Design review of the part built by this model. Coordinates are the model's own, in mm. Face numbers are marked on the shaded views. Coordinates: 2 decimals unless noted, no trailing zeros. Loops run counter-clockwise (first coordinate to the right, second up) from the corner with the lowest first, then second, coordinate; pieces in that order, holes last. Notation, with made-up numbers: (-20, 73.5) -> (13, 73.5) arc R24 cw to (13, 93.5) -> close; hole circle Ø1 at (-16.5, 68). An arc over 180 degrees is marked (long way). Answer in a Markdown table with one row per item.
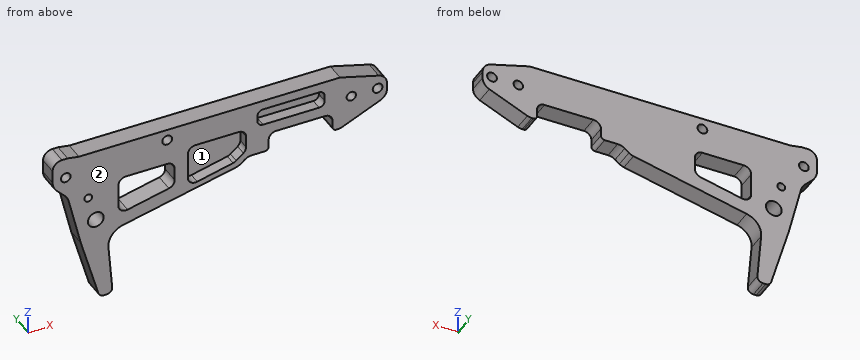
```python
from build123d import *

# Parameters (mm, degrees)
SKETCH1_R           = 2.6
SKETCH1_R_2         = 2.1
SKETCH1_R_3         = 4.2
SKETCH1_R_4         = 2.5
BOSS_EXTRUDE1_DEPTH = 10
FILLET2_R           = 6
FILLET3_R           = 3
CUT_EXTRUDE1_DEPTH  = 11
SKETCH7_R           = 2.6
CUT_EXTRUDE4_DEPTH  = 11
FILLET8_R           = 5
FILLET9_R           = 4
SKETCH10_W          = 34
SKETCH10_H          = 10
CUT_EXTRUDE6_DEPTH  = 11
FILLET10_R          = 4
CUT_EXTRUDE7_DEPTH  = 6
FILLET14_R          = 6
FILLET15_R          = 2
FILLET16_R          = 10
FILLET17_R          = 8
FILLET18_R          = 4
SKETCH13_W          = 35.854861743
SKETCH13_H          = 9
CUT_EXTRUDE8_DEPTH  = 6
FILLET19_R          = 3


with BuildPart() as part:
    # Sketch1 → Boss-Extrude1 (new body)
    with BuildSketch(Plane(origin=(0, 0, 0), x_dir=(1, 0, 0), z_dir=(0, 1, 0))):
        Polygon((164, 19), (139, 30), (90, 30), (85, 34), (15, 50), (18, 86), (11, 86), (1, 51), (-6, 22), (-14, 14), (-14, 2), (-14, -1), (-6, -1), (0, 0), (139, 0), (164, 7), align=None)
        with Locations((-7, 10)):
            Circle(SKETCH1_R, mode=Mode.SUBTRACT)
        with Locations((159, 13)):
            Circle(SKETCH1_R, mode=Mode.SUBTRACT)
        with Locations((5, 26)):
            Circle(SKETCH1_R_2, mode=Mode.SUBTRACT)
        with Locations((9, 40)):
            Circle(SKETCH1_R_3, mode=Mode.SUBTRACT)
        with Locations((145, 13)):
            Circle(SKETCH1_R_4, mode=Mode.SUBTRACT)
    extrude(amount=BOSS_EXTRUDE1_DEPTH)

    # Fillet2
    fillet2_edges = [part.edges().sort_by_distance(p)[0] for p in [
        (139, 5, -30),
        (164, 5, -19),
        (164, 5, -7),
    ]]
    fillet(fillet2_edges, radius=FILLET2_R)

    # Fillet3
    fillet3_edges = [part.edges().sort_by_distance(p)[0] for p in [
        (11, 5, -86),
        (18, 5, -86),
    ]]
    fillet(fillet3_edges, radius=FILLET3_R)

    # Sketch4 → Cut-Extrude1 (cut, through all)
    with BuildSketch(Plane(origin=(0, 10, 0), x_dir=(1, 0, 0), z_dir=(0, 1, 0))):
        Polygon((21, 41), (21, 20), (51, 20), (51, 34), align=None)
    extrude(amount=-CUT_EXTRUDE1_DEPTH, mode=Mode.SUBTRACT)

    # Sketch7 → Cut-Extrude4 (cut, through all)
    with BuildSketch(Plane(origin=(0, 10, 0), x_dir=(1, 0, 0), z_dir=(0, 1, 0))):
        with Locations((47, 6)):
            Circle(SKETCH7_R)
    extrude(amount=-CUT_EXTRUDE4_DEPTH, mode=Mode.SUBTRACT)

    # Fillet8
    fillet8_edges = [part.edges().sort_by_distance(p)[0] for p in [
        (-14, 5, 1),
    ]]
    fillet(fillet8_edges, radius=FILLET8_R)

    # Fillet9
    fillet9_edges = [part.edges().sort_by_distance(p)[0] for p in [
        (21, 5, -41),
        (51, 5, -34),
        (51, 5, -20),
        (21, 5, -20),
    ]]
    fillet(fillet9_edges, radius=FILLET9_R)

    # Sketch10 → Cut-Extrude6 (cut, through all)
    with BuildSketch(Plane(origin=(0, 10, 0), x_dir=(1, 0, 0), z_dir=(0, 1, 0))):
        with Locations((118, 25)):
            Rectangle(SKETCH10_W, SKETCH10_H)
    extrude(amount=-CUT_EXTRUDE6_DEPTH, mode=Mode.SUBTRACT)

    # Fillet10
    fillet10_edges = [part.edges().sort_by_distance(p)[0] for p in [
        (135, 5, -20),
        (101, 5, -20),
    ]]
    fillet(fillet10_edges, radius=FILLET10_R)

    # Sketch12 → Cut-Extrude7 (cut)
    with BuildSketch(Plane(origin=(0, 0, 0), x_dir=(1, 0, 0), z_dir=(0, 1, 0))):
        Polygon((58, 37), (83, 31.034746853), (89, 26.034746853), (89, 14), (58, 14), align=None)
    extrude(amount=CUT_EXTRUDE7_DEPTH, mode=Mode.SUBTRACT)

    # Fillet14
    fillet14_edges = [part.edges().sort_by_distance(p)[0] for p in [
        (85, 5, -34),
        (90, 5, -30),
    ]]
    fillet(fillet14_edges, radius=FILLET14_R)

    # Fillet15
    fillet15_edges = [part.edges().sort_by_distance(p)[0] for p in [
        (101, 5, -30),
        (135, 5, -30),
    ]]
    fillet(fillet15_edges, radius=FILLET15_R)

    # Fillet16
    fillet16_edges = [part.edges().sort_by_distance(p)[0] for p in [
        (15, 5, -50),
    ]]
    fillet(fillet16_edges, radius=FILLET16_R)

    # Fillet17
    fillet17_edges = [part.edges().sort_by_distance(p)[0] for p in [
        (-14, 5, -14),
        (-6, 5, -22),
    ]]
    fillet(fillet17_edges, radius=FILLET17_R)

    # Fillet18
    fillet18_edges = [part.edges().sort_by_distance(p)[0] for p in [
        (58, 3, -37),
        (58, 3, -14),
        (89, 3, -14),
        (89, 3, -26.034746853),
        (83, 3, -31.034746853),
    ]]
    fillet(fillet18_edges, radius=FILLET18_R)

    # Sketch13 → Cut-Extrude8 (cut)
    with BuildSketch(Plane.XZ):
        with Locations((112.927430872, -9.5)):
            Rectangle(SKETCH13_W, SKETCH13_H)
    extrude(amount=-CUT_EXTRUDE8_DEPTH, mode=Mode.SUBTRACT)

    # Fillet19
    fillet19_edges = [part.edges().sort_by_distance(p)[0] for p in [
        (130.854861743, 3, -5),
        (130.854861743, 3, -14),
        (95, 3, -14),
        (95, 3, -5),
    ]]
    fillet(fillet19_edges, radius=FILLET19_R)


solid = part.part
```
(1) To check wall thickness, follow probe 1 along X at (y, z) = (5.25, -26); probe 2 along X at (y, z) = (2.25, -13); probe 3 along X at (y, z) = (4.5, -10). State the ranges of each line that lie inside material, in increasing order.
Evaluation:
| item | result |
|---|---|
| probe 1 | x = -5.03 to 2.9, 7.1 to 21, 51 to 58, 88.55 to 101, 135 to 148.09 |
| probe 2 | x = -13.66 to 95.76, 130.09 to 142.5, 147.5 to 156.4, 161.6 to 164 |
| probe 3 | x = -14 to -9.6, -4.4 to 95, 130.85 to 163.8 |
(2) Take a section at A-A on y = 2.5. Count the separate pieces of the cut face and the enclosed holes in it, and give its area (3 significant figures).
Evaluation:
| item | result |
|---|---|
| separate pieces | 1 |
| enclosed holes | 9 |
| area | 4,700 mm² |
(3) For pin 1 (3 mm diameter, centred on y = 3, z = -20, fed in from -X); pin 2 (5 mm diameter, centred on x = 107, y = 4, fed in from -Z); pin 3 (1 mm diameter, centred on y = 9, z = -51.5, fed in from +X); pin 4 (7 mm diameter, centred on x = 159, z = -13, fed in from -Y), all flat-tipped, find the tip position at first contact; note any pin that passes through.
Evaluation:
| item | result |
|---|---|
| pin 1 | stops at x = -9.5 |
| pin 2 | stops at z = -20.03 |
| pin 3 | stops at x = 18.37 |
| pin 4 | stops at y = 0 |
(4) Take a section at C-C on z = -68.5. Give the boundary of the cut face in (x, y).
Evaluation:
| item | result |
|---|---|
| outline | (6, 0) -> (16.54, 0) -> (16.54, 10) -> (6, 10) -> close |
(5) Draft analysis for pull direction X (two halves, no side actions). For the marked faces 1 and 2, state which applies: pulls with the +X half, pulls with the -X half, needs draft (parallel to the pull), parting line crosses it, or undercut.
Evaluation:
| item | result |
|---|---|
| face 1 | undercut |
| face 2 | needs draft |
(6) Take a section at B-B on x = 108. Give the boundary of the cut face in (y, z), and give its area (3 significant figures).
Evaluation:
| item | result |
|---|---|
| outline | (0, -20) -> (10, -20) -> (10, 0) -> (0, 0) -> (0, -5) -> (6, -5) -> (6, -14) -> (0, -14) -> close |
| area | 146 mm² |
